```python
from build123d import *

# Parameters (mm, degrees)
SKETCH1_R           = 6.35
BOSS_EXTRUDE1_DEPTH = 3


with BuildPart() as part:
    # Sketch1 → Boss-Extrude1 (new body)
    with BuildSketch(Plane(origin=(0, 0, 0), x_dir=(1, 0, 0), z_dir=(0, 1, 0))):
        Polygon((48, -4), (41.080632081, -4), (41.080632081, 4), (48, 4), (48, 35), (35, 48), (4, 48), (4, 41.080632081), (-4, 41.080632081), (-4, 48), (-35, 48), (-48, 35), (-48, 4), (-41.08063208, 4), (-41.08063208, -4), (-48, -4), (-48, -35), (-35, -48), (-4, -48), (-4, -41.080632081), (4, -41.080632081), (4, -48), (35, -48), (48, -35), align=None)
        Circle(SKETCH1_R, mode=Mode.SUBTRACT)
        with BuildLine():
            Line((-30.337295283, 34.57993597), (-8.42006403, 12.662704717))
            ThreePointArc((-8.42006403, 12.662704717), (-4.959980102, 11.974451232), (-3, 14.907768748))
            Line((-3, 14.907768748), (-3, 30.475))
            ThreePointArc((-3, 30.475), (-5.789807909, 37.210192091), (-12.525, 40))
            Line((-12.525, 40), (-28.092231252, 40))
            ThreePointArc((-28.092231252, 40), (-31.025548768, 38.040019898), (-30.337295283, 34.57993597))
        make_face(mode=Mode.SUBTRACT)
        with BuildLine():
            Line((3, 14.907768748), (3, 30.475))
            ThreePointArc((3, 30.475), (5.789807909, 37.210192091), (12.525, 40))
            Line((12.525, 40), (28.092231252, 40))
            ThreePointArc((28.092231252, 40), (31.025548768, 38.040019898), (30.337295283, 34.57993597))
            Line((30.337295283, 34.57993597), (8.42006403, 12.662704717))
            ThreePointArc((8.42006403, 12.662704717), (4.959980102, 11.974451232), (3, 14.907768748))
        make_face(mode=Mode.SUBTRACT)
        with BuildLine():
            Line((12.662704717, 8.42006403), (34.57993597, 30.337295283))
            ThreePointArc((34.57993597, 30.337295283), (38.040019898, 31.025548768), (40, 28.092231252))
            Line((40, 28.092231252), (40, 6.175))
            ThreePointArc((40, 6.175), (39.07006403, 3.92993597), (36.825, 3))
            Line((36.825, 3), (14.907768748, 3))
            ThreePointArc((14.907768748, 3), (11.974451232, 4.959980102), (12.662704717, 8.42006403))
        make_face(mode=Mode.SUBTRACT)
        with BuildLine():
            Line((40, -6.175), (40, -28.092231252))
            ThreePointArc((40, -28.092231252), (38.040019898, -31.025548768), (34.57993597, -30.337295283))
            Line((34.57993597, -30.337295283), (12.662704717, -8.42006403))
            ThreePointArc((12.662704717, -8.42006403), (11.974451232, -4.959980102), (14.907768747, -3))
            Line((14.907768747, -3), (36.825, -3))
            ThreePointArc((36.825, -3), (39.07006403, -3.92993597), (40, -6.175))
        make_face(mode=Mode.SUBTRACT)
        with BuildLine():
            Line((30.337295283, -34.57993597), (8.42006403, -12.662704717))
            ThreePointArc((8.42006403, -12.662704717), (4.959980102, -11.974451232), (3, -14.907768748))
            Line((3, -14.907768748), (3, -30.475))
            ThreePointArc((3, -30.475), (5.789807909, -37.210192091), (12.525, -40))
            Line((12.525, -40), (28.092231252, -40))
            ThreePointArc((28.092231252, -40), (31.025548768, -38.040019898), (30.337295283, -34.57993597))
        make_face(mode=Mode.SUBTRACT)
        with BuildLine():
            Line((-3, -14.907768748), (-3, -30.475))
            ThreePointArc((-3, -30.475), (-5.789807909, -37.210192091), (-12.525, -40))
            Line((-12.525, -40), (-28.092231252, -40))
            ThreePointArc((-28.092231252, -40), (-31.025548768, -38.040019898), (-30.337295283, -34.57993597))
            Line((-30.337295283, -34.57993597), (-8.42006403, -12.662704717))
            ThreePointArc((-8.42006403, -12.662704717), (-4.959980102, -11.974451232), (-3, -14.907768748))
        make_face(mode=Mode.SUBTRACT)
        with BuildLine():
            Line((-34.57993597, -30.337295283), (-12.662704717, -8.42006403))
            ThreePointArc((-12.662704717, -8.42006403), (-11.974451232, -4.959980102), (-14.907768747, -3))
            Line((-14.907768747, -3), (-36.825, -3))
            ThreePointArc((-36.825, -3), (-39.07006403, -3.92993597), (-40, -6.175))
            Line((-40, -6.175), (-40, -28.092231252))
            ThreePointArc((-40, -28.092231252), (-38.040019898, -31.025548768), (-34.57993597, -30.337295283))
        make_face(mode=Mode.SUBTRACT)
        with BuildLine():
            Line((-36.825, 3), (-14.907768748, 3))
            ThreePointArc((-14.907768748, 3), (-11.974451232, 4.959980102), (-12.662704717, 8.42006403))
            Line((-12.662704717, 8.42006403), (-34.57993597, 30.337295283))
            ThreePointArc((-34.57993597, 30.337295283), (-38.040019898, 31.025548768), (-40, 28.092231252))
            Line((-40, 28.092231252), (-40, 6.175))
            ThreePointArc((-40, 6.175), (-39.07006403, 3.92993597), (-36.825, 3))
        make_face(mode=Mode.SUBTRACT)
    extrude(amount=BOSS_EXTRUDE1_DEPTH)


solid = part.part
```
Geometry check sheet. Reference: the model listing, model coordinates, mm. A direction names the side the tool comes from. Round coordinates to 2 decimals unless told otherwise and drop trailing zeros. Write each loop counter-clockwise with the first axis right and the second up, starting at its lowest first coordinate (ties: lowest second). Pieces come first, ordered by that corner, then holes. Notation, with made-up numbers: (81.5, 2) -> (135.5, 2) arc R14 cw to (135.5, 23) -> close; hole circle Ø5 at (0, 62.25). An arc over 180 degrees is marked (long way). Put each result on its own line as item: value.
1) Cross-section at B-B, the plane x = 0. Enter the section's corners in (y, z).
Recorded:
outline: (0, -41.08) -> (3, -41.08) -> (3, -6.35) -> (0, -6.35) -> close; (0, 6.35) -> (3, 6.35) -> (3, 41.08) -> (0, 41.08) -> close
2) Release check for a two-part mould opening along Z. For faces 1 (the face through (-48, 1, -20)), 2 (the face through (-19.53, 1.48, -23.77)), 3 (the face through (0, 1, 41.081)) record: pulls with the +Z half, pulls with the -Z half, needs draft (parallel to the pull), parting line crosses it, or undercut.
Recorded:
face 1: needs draft
face 2: undercut
face 3: pulls with the +Z half
3) Depth check by flat-ended pin: P1, Ø0.9, axis at x = -44, y = 1, coming from the +Z side; P2, Ø0.9, axis at x = -1.5, y = 1.5, coming from the +Z side; P3, Ø16.5, axis at x = 0, z = 0, coming from the +Y side; P4, Ø1.5, axis at y = 2, z = 44, coming from the -X side. Enter the tip coordinate at first touch or a pass-through.
Recorded:
P1: stops at z = 39.45
P2: stops at z = 41.08
P3: stops at y = 3
P4: stops at x = -39.75
4) Cross-section at A-A, the plane z = 0. Enter the section's corners in (x, y).
Recorded:
outline: (-41.08, 0) -> (-6.35, 0) -> (-6.35, 3) -> (-41.08, 3) -> close; (6.35, 0) -> (41.08, 0) -> (41.08, 3) -> (6.35, 3) -> close
5) Cross-section at C-C, the plane x = 38. Enter the section's corners in (y, z).
Recorded:
outline: (0, -45) -> (3, -45) -> (3, -31.04) -> (0, -31.04) -> close; (0, -3.23) -> (3, -3.23) -> (3, 3.23) -> (0, 3.23) -> close; (0, 31.04) -> (3, 31.04) -> (3, 45) -> (0, 45) -> close
6) Thickness scan on probe 1 along X at (y, z) = (0.9, 0); probe 2 along Z at (x, y) = (-5, 2.05). Record the ranges inside material, lowest first. Write a range as from..to.
Recorded:
probe 1: x = -41.08..-6.35, 6.35..41.08
probe 2: z = -48..-36.31, -11.96..-3.91, 3.91..11.96, 36.31..48
7) Access from +Z, -Z, +X, -X, +Y, -Y to the whole of each face (thin tool, end or side, straight path). Record for faces 4 (the face through (41.081, 1, 0)), 5 (the face through (5.72, 1.48, 37.14)), 6 (the face through (4, 1, -45)).
Recorded:
face 4: +X, +Y, -Y
face 5: +Y, -Y
face 6: -Z, +Y, -Y
8) Cross-section at D-D, the plane y = 1.1. Give the number of separate pieces and of enclosed holes in the cut face, plus the area to 3 significant figures.
Recorded:
separate pieces: 1
enclosed holes: 9
area: 4,520 mm2
